Design review of the part shown in the three views and the two pictorial views. Dimensions are in mm from the part's minimum x, y and z. A direction names the side the tool comes from. Round coordinates to 2 decimals unless told otherwise and drop trailing zeros. Write each loop counter-clockwise with the first axis right and the second up, starting at its lowest first coordinate (ties: lowest second). Pieces come first, ordered by that corner, then holes. Notation, with made-up numbers: (-36, 78.5) - (-30, 78.5) arc R19 cw to (-30, 88.5) - close; hole circle Ø4 at (-12, 17.25). An arc over 180 degrees is marked (long way). Use one line per item in the form item = value.
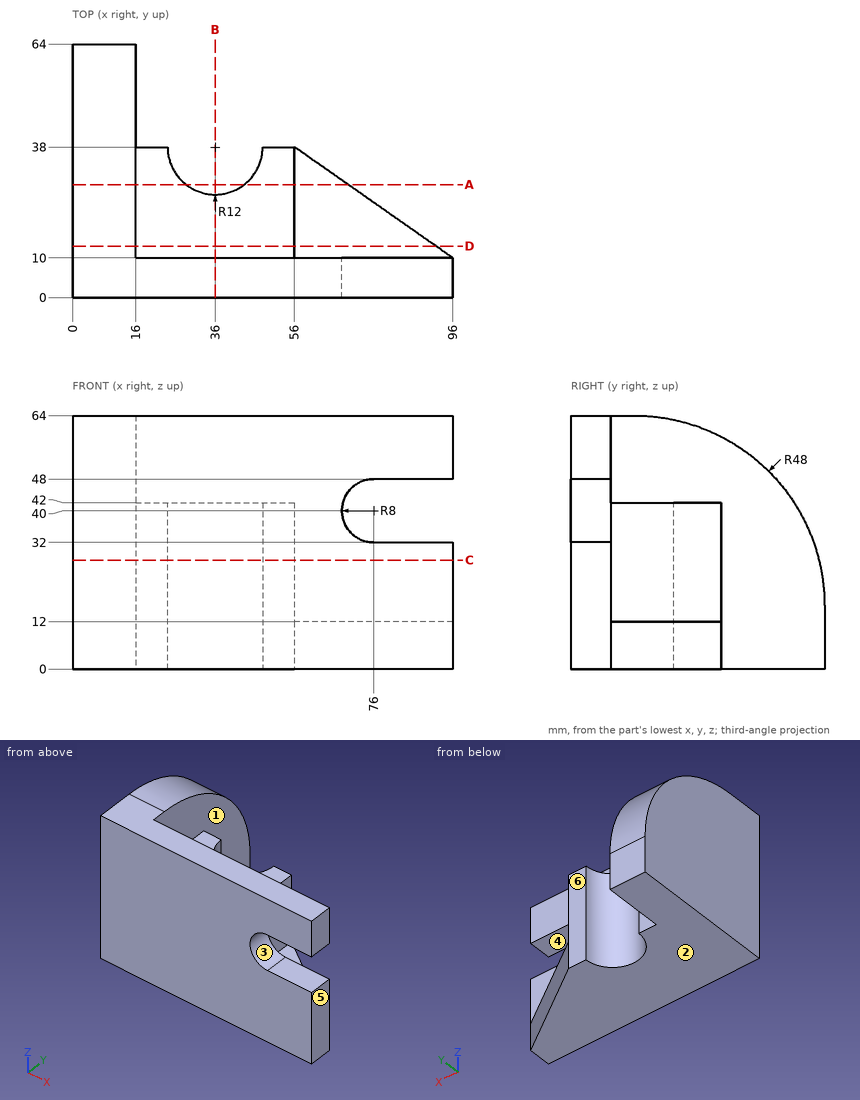
Q1. We need section B-B on x = 36. Write out the cut boundary in (y, z), then the cut area to 3 significant figures.
Calculated:
outline = (0, 0) - (26, 0) - (26, 42) - (10, 42) - (10, 64) - (0, 64) - close
area = 1,310 mm2
Q2. Draft analysis for pull direction Z (two halves, no side actions). For the marked faces 1, 2 and 3, state which applies: released by +Z, released by -Z, zero draft, split by the parting line, or undercut.
Calculated:
face_1 = zero draft
face_2 = released by -Z
face_3 = undercut
Q3. Machinability: for the marked faces 4, 5 and 6, which of the approach directions +Z, -Z, +X, -X, +Y, -Y give a long, thin tool a straight path to every point of the face, cutting with its end or side? Answer none if there is none.
Calculated:
face_4 = +X, +Y, -Y
face_5 = +Z, -Z, +X, +Y, -Y
face_6 = +Z, -Z, +X, +Y
Q4. We need section A-A on y = 28.5. Write out the cut boundary in (x, z).
Calculated:
outline = (0, 0) - (28.67, 0) - (28.67, 42) - (16, 42) - (16, 62.34) - (0, 62.34) - close; (43.33, 0) - (69.57, 0) - (69.57, 12) - (56, 12) - (56, 42) - (43.33, 42) - close
Q5. To check wall thickness, follow line 1 along Y through (x, z) = (60, 13.5); line 2 along Z through (x, y) = (45, 14); line 3 along X through (y, z) = (38, 44). State the ranges of each line that lie inside material, in increasing order. Write a range as from..to.
Calculated:
line_1 = 0..10
line_2 = 0..42
line_3 = 0..16
Q6. We need section C-C on z = 27.5. Write out the cut boundary in (x, y), then the cut area to 3 significant figures.
Calculated:
outline = (0, 0) - (96, 0) - (96, 10) - (56, 10) - (56, 38) - (48, 38) arc R12 cw to (24, 38) - (16, 38) - (16, 62.6) - (0, 62.6) - close
area = 2,700 mm2
Q7. For P1, Ø14, axis at x = 81, y = 25.5, coming from the +Z side; P2, Ø8, axis at x = 11.5, y = 29, coming from the +Z side; P3, Ø2.5, axis at x = 51.5, z = 26.5, coming from the +Y side, all flat-tipped, find the tip position at first contact; note any pin that passes through.
Calculated:
P1 = 12
P2 = 63.15
P3 = 38
Q8. We need section D-D on y = 13. Write out the cut boundary in (x, z), then the cut area to 3 significant figures.
Calculated:
outline = (0, 0) - (91.71, 0) - (91.71, 12) - (56, 12) - (56, 42) - (16, 42) - (16, 64) - (0, 64) - close
area = 3,130 mm2
